Design review of the part built by this model. Coordinates are the model's own, in mm. Face numbers are marked on the shaded views. A direction names the side the tool comes from. Round coordinates to 2 decimals unless told otherwise and drop trailing zeros. Write each loop counter-clockwise with the first axis right and the second up, starting at its lowest first coordinate (ties: lowest second). Pieces come first, ordered by that corner, then holes. Notation, with made-up numbers: (-32, 51.25) -> (26, 51.25) arc R27 cw to (26, 90.25) -> close; hole circle Ø8 at (70, -30). An arc over 180 degrees is marked (long way). One line per question, with ' | ' between items. Start each with the question number.
1) For the marked faces 1 and 2, list the 3-axis set-ups (+Z, -Z, +X, -X, +Y, -Y) from which the entire face can be reached by the end or side of a thin tool; tool diameter is ignored.
2) Consider section A-A (z = -14). Give the boundary of the cut face in (x, y).
3) Mouldability with a two-part tool opening along X and no side actions: class the marked faces 3, 4 and 5 as +X half, -X half, draft (parallel to the pull), parting line (faces both ways), or undercut.
4) Consider section C-C (y = -25). Give the boundary of the cut face in (x, z).
5) Consider section B-B (x = -42.5). Give the boundary of the cut face in (y, z), then the cut area to 3 significant figures.
6) For probe 1 along X at (y, z) = (-40.5, -4); probe 2 along Y at (x, z) = (-77, -4); probe 3 along X at (y, z) = (-63.5, -14.5), list the stretches that pass through material, from the lowest coordinate up.
7) Consider section D-D (x = 62). Give the boundary of the cut face in (y, z).
8) Insertion check: pin 1 Ø4 at (y, z) = (3.5, -28.5) entering from +X; pin 2 Ø25 at (x, y) = (17, -3) entering from +Z; pin 3 Ø1 at (y, z) = (9.5, -21) entering from -X. Each pin has a flat end and moves straight along its axis. Give the tip position at first contact, or say it passes through.
```python
from build123d import *

# Parameters (mm, degrees)
F0_W     = 177
F0_H     = 90.5
F1_DEPTH = 46
F2_W     = 84
F2_H     = 84
F3_DEPTH = 44
F4_R     = 20


with BuildPart() as f1:
    # F0 (on Top) → F1 (new body)
    with BuildSketch(Plane.XY):
        with Locations((-11.741341, -23.917309)):
            Rectangle(F0_W, F0_H)
    extrude(amount=-F1_DEPTH)

    # F2 (on face) → F3 (cut)
    with BuildSketch(Plane.XY):
        with Locations((-54.741341, -23.667309)):
            Rectangle(F2_W, F2_H)
        with Locations((31.258659, -23.667309)):
            Rectangle(F2_W, F2_H)
    extrude(amount=-F3_DEPTH, mode=Mode.SUBTRACT)

    # F4
    f4_edges = [f1.edges().sort_by_distance(p)[0] for p in [
        (-96.741341, 18.332691, -22),
        (-96.741341, -65.667309, -22),
        (-12.741341, -65.667309, -22),
        (-12.741341, 18.332691, -22),
        (-10.741341, 18.332691, -22),
        (-10.741341, -65.667309, -22),
        (73.258659, 18.332691, -22),
        (73.258659, -65.667309, -22),
        (76.758659, 21.332691, -23),
        (-100.241341, 21.332691, -23),
        (-100.241341, -69.167309, -23),
        (76.758659, -69.167309, -23),
    ]]
    fillet(f4_edges, radius=F4_R)


solid = f1.part
```
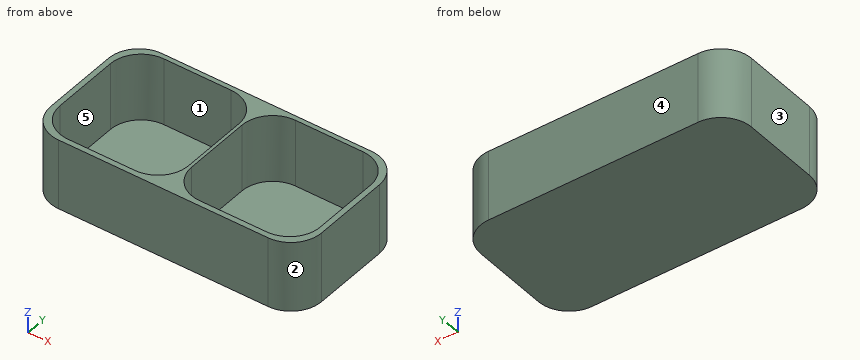
From the geometry:
1) face 1: +Z | face 2: +Z, -Z, +X, -Y
2) outline: (-100.24, -49.17) arc R20 ccw to (-80.24, -69.17) -> (56.76, -69.17) arc R20 ccw to (76.76, -49.17) -> (76.76, 1.33) arc R20 ccw to (56.76, 21.33) -> (-80.24, 21.33) arc R20 ccw to (-100.24, 1.33) -> close; hole (-96.74, -45.67) arc R20 ccw to (-76.74, -65.67) -> (-32.74, -65.67) arc R20 ccw to (-12.74, -45.67) -> (-12.74, -1.67) arc R20 ccw to (-32.74, 18.33) -> (-76.74, 18.33) arc R20 ccw to (-96.74, -1.67) -> close; hole (-10.74, -45.67) arc R20 ccw to (9.26, -65.67) -> (53.26, -65.67) arc R20 ccw to (73.26, -45.67) -> (73.26, -1.67) arc R20 ccw to (53.26, 18.33) -> (9.26, 18.33) arc R20 ccw to (-10.74, -1.67) -> close
3) face 3: -X half | face 4: draft | face 5: undercut
4) outline: (-100.24, -46) -> (76.76, -46) -> (76.76, 0) -> (73.26, 0) -> (73.26, -44) -> (-10.74, -44) -> (-10.74, 0) -> (-12.74, 0) -> (-12.74, -44) -> (-96.74, -44) -> (-96.74, 0) -> (-100.24, 0) -> close
5) outline: (-69.17, -46) -> (21.33, -46) -> (21.33, 0) -> (18.33, 0) -> (18.33, -44) -> (-65.67, -44) -> (-65.67, 0) -> (-69.17, 0) -> close | area: 467 mm2
6) probe 1: x = -100.24 to -96.74, -12.74 to -10.74, 73.26 to 76.76 | probe 2: y = -69.17 to -65.67, 18.33 to 21.33 | probe 3: x = -94.19 to -85.8, -23.69 to 0.2, 62.31 to 70.71
7) outline: (-68.47, -46) -> (20.63, -46) -> (20.63, 0) -> (16.32, 0) -> (16.32, -44) -> (-63.66, -44) -> (-63.66, 0) -> (-68.47, 0) -> close
8) pin 1: stops at x = 76.76 | pin 2: stops at z = -44 | pin 3: stops at x = -98.71
